Work out the finished part from the listing and answer in its coordinate system (mm). A direction names the side the tool comes from. Give positions to 0.01 mm unless a question says otherwise; leave off trailing zeros. Order: outer loops, then holes, each group sorted by start corner. A loop starts at its lowest first (then second) coordinate and runs counter-clockwise, first axis right, second up. Notation, with made-up numbers: M -38,12.5 L 20,12.5 A23 ccw 20,30.5 Z; hole C -31,1.25 d11. An arc over 180 degrees is marked long. One line per item, written item: value.
from build123d import *

# Parameters (mm, degrees)
SKETCH2_R          = 5
CUT_EXTRUDE1_DEPTH = 35.5
CIRPATTERN1_COUNT  = 4


with BuildPart() as part:
    # Sketch1 → Revolve1 (revolve)
    with BuildSketch(Plane.XY):
        Polygon((11.880841121, 0), (22.5, 0), (31.753664233, 42), (25.609760166, 42), (19, 12), (11, 12), (11, 0), align=None)
    revolve(axis=Axis((0, 0, 0), (0, 1, 0)))

    # Sketch2 → Cut-Extrude1 (cut, symmetric)
    with BuildSketch(Plane.XY):
        with Locations((0, 42)):
            Circle(SKETCH2_R)
    cut_extrude1 = extrude(amount=CUT_EXTRUDE1_DEPTH, both=True, mode=Mode.SUBTRACT)

    # CirPattern1: Cut-Extrude1 ×4 about axis
    cirpattern1_axis = Axis((0, 0, 0), (0, 1, 0))
    for i in range(1, CIRPATTERN1_COUNT):
        add(cut_extrude1.rotate(cirpattern1_axis, i * 360 / CIRPATTERN1_COUNT), mode=Mode.SUBTRACT)


solid = part.part
(1) Find the intervals of material crossed by probe 1 along X at (y, z) = (6.25, 0); probe 2 along Z at (x, y) = (0, 2); probe 3 along Z at (x, y) = (0, 8.75), in increasing order. Write a range as from..to.
Findings:
probe 1: x = -23.88..-11, 11..23.88
probe 2: z = -22.94..-11, 11..22.94
probe 3: z = -24.43..-11, 11..24.43
(2) Section A-A, the plane z = 0 is taken. Give the vertices of the cut face in (x, y).
Findings:
outline: M -30.65,37 L -22.5,0 L -11,0 L -11,12 L -19,12 L -24.51,37 Z; M 11,0 L 22.5,0 L 30.65,37 L 24.51,37 L 19,12 L 11,12 Z
(3) Determine the mould class of faces 1 (the cylindrical face through (-28, 37, 0)), 2 (the flat face through (-19, 42, -20)), 3 (the conical face through (12.073, 16.627, 23.211)) for opening direction Z: pulls with the +Z half, pulls with the -Z half, needs draft (parallel to the pull), parting line crosses it, or undercut.
Findings:
face 1: undercut
face 2: needs draft
face 3: parting line crosses it
(4) Section C-C, the plane y = 25.5 is taken. Give the vertices of the cut face in (x, z), then the cut area to 3 significant figures.
Findings:
outline: C 0,0 d56.24; hole C 0,0 d43.95
area: 967 mm^2
(5) Which of the six approach directions +Z, -Z, +X, -X, +Y, -Y give full straight-line access (tool end or side, diameter ignored) to faces 4 (the flat face through (19, 42, -18)), 5 (the flat face through (8, 12, 8))?
Findings:
face 4: +Z, -Z, +X, -X, +Y
face 5: +Y
(6) Section B-B, the plane x = 0 is taken. Give the vertices of the cut face in (y, z), then the cut area to 3 significant figures.
Findings:
outline: M 0,-22.5 L 37,-30.65 L 37,-24.51 L 12,-19 L 12,-11 L 0,-11 Z; M 0,11 L 12,11 L 12,19 L 37,24.51 L 37,30.65 L 0,22.5 Z
area: 615 mm^2
(7) Section D-D, the plane y = 35.5 is taken. Give the vertices of the cut face in (x, z), then the cut area to 3 significant figures.
Findings:
outline: C 0,0 d60.64; hole C 0,0 d48.36
area: 1,050 mm^2
(8) Given P1, Ø1, axis at x = -10.5, y = 30, coming from the +Z side; P2, Ø6, axis at y = 13.5, z = -13.5, coming from the -X side; P3, Ø8, axis at x = 6.5, y = 33, coming from the -Z side, each flat-ended and moving along its own axis, determine where each tip first touches the part or whether it passes through.
Findings:
P1: stops at z = 27.37
P2: stops at x = -23.39
P3: stops at z = -30.2
